```python
from build123d import *

# Parameters (mm, degrees)
RESSALTO_EXTRUS_O1_DEPTH = 22.5
CHANFRO1_SIZE            = 9
CORTE_EXTRUS_O1_REACH    = 24.5
ESBO_O3_W                = 1139.230904301
ESBO_O3_H                = 709.798033895
CORTE_EXTRUS_O5_DEPTH    = 1.5
ESBO_O5_R                = 3
CORTE_EXTRUS_O6_DEPTH    = 22
CORTE_EXTRUS_O8_DEPTH    = 10
CORTE_EXTRUS_O12_DEPTH   = 15
ESBO_O13_R               = 10.5
CORTE_EXTRUS_O13_DEPTH   = 5


with BuildPart() as part:
    # Esboço1 → Ressalto-extrusão1 (new body, symmetric)
    with BuildSketch(Plane.XY):
        with BuildLine():
            Line((-57.319579452, -8.082215343), (57.319579452, -8.082215343))
            Line((57.319579452, -8.082215343), (70, 2.557920862))
            Line((70, 2.557920862), (70, 117.296691049))
            ThreePointArc((70, 117.296691049), (70.546863139, 120.39810603), (72.121492792, 123.125444592))
            Line((72.121492792, 123.125444592), (112.878507208, 171.697762944))
            ThreePointArc((112.878507208, 171.697762944), (114.453136861, 174.425101506), (115, 177.526516487))
            Line((115, 177.526516487), (115, 237.712528581))
            ThreePointArc((115, 237.712528581), (114.396926208, 241.132730014), (112.660444431, 244.140404678))
            Line((112.660444431, 244.140404678), (75.567830361, 288.345660754))
            ThreePointArc((75.567830361, 288.345660754), (72.133568548, 290.980862527), (67.90738593, 291.917784657))
            Line((67.90738593, 291.917784657), (-67.90738593, 291.917784657))
            ThreePointArc((-67.90738593, 291.917784657), (-72.133568548, 290.980862527), (-75.567830361, 288.345660754))
            Line((-75.567830361, 288.345660754), (-112.660444431, 244.140404678))
            ThreePointArc((-112.660444431, 244.140404678), (-114.396926208, 241.132730014), (-115, 237.712528581))
            Line((-115, 237.712528581), (-115, 177.526516487))
            ThreePointArc((-115, 177.526516487), (-114.453136861, 174.425101506), (-112.878507208, 171.697762944))
            Line((-112.878507208, 171.697762944), (-72.121492792, 123.125444592))
            ThreePointArc((-72.121492792, 123.125444592), (-70.546863139, 120.39810603), (-70, 117.296691049))
            Line((-70, 117.296691049), (-70, 2.557920862))
            Line((-70, 2.557920862), (-57.319579452, -8.082215343))
        make_face()
        Polygon((-90, 175.546696324), (-90, 238.538123078), (-61.99113828, 271.917784657), (61.99113828, 271.917784657), (90, 238.538123078), (90, 175.546696324), (45, 121.917784657), (45, 11.917784657), (-45, 11.917784657), (-45, 121.917784657), align=None, mode=Mode.SUBTRACT)
    extrude(amount=RESSALTO_EXTRUS_O1_DEPTH, both=True)

    # Chanfro1
    chanfro1_edges = [part.edges().sort_by_distance(p)[0] for p in [
        (0, -8.082215343, 22.5),
        (63.659789726, -2.76214724, 22.5),
        (70, 59.927305955, 22.5),
        (70.546863139, 120.39810603, 22.5),
        (92.5, 147.411603768, 22.5),
        (114.453136861, 174.425101506, 22.5),
        (115, 207.619522534, 22.5),
        (114.396926208, 241.132730014, 22.5),
        (94.114137396, 266.243032716, 22.5),
        (72.133568548, 290.980862527, 22.5),
        (0, 291.917784657, 22.5),
        (-72.133568548, 290.980862527, 22.5),
        (-94.114137396, 266.243032716, 22.5),
        (-114.396926208, 241.132730014, 22.5),
        (-115, 207.619522534, 22.5),
        (-114.453136861, 174.425101506, 22.5),
        (-92.5, 147.411603768, 22.5),
        (-70.546863139, 120.39810603, 22.5),
        (-70, 59.927305955, 22.5),
        (-63.659789726, -2.76214724, 22.5),
    ]]
    chamfer(chanfro1_edges, length=CHANFRO1_SIZE)

    # Esboço3 → Corte-extrusão1 (cut, up to next)
    with BuildSketch(Plane.XY, mode=Mode.PRIVATE) as corte_extrus_o1_sk1:
        with Locations((-153.157436203, 152.53565808)):
            Rectangle(ESBO_O3_W, ESBO_O3_H)
    corte_extrus_o1_tool1 = extrude(corte_extrus_o1_sk1.sketch, amount=-CORTE_EXTRUS_O1_REACH, mode=Mode.PRIVATE) & part.part
    add(corte_extrus_o1_tool1.solids().sort_by_distance((-153.157436, 152.535658, 0))[0], mode=Mode.SUBTRACT)

    # Esboço4 → Corte-extrusão5 (cut)
    with BuildSketch(Plane.XY.offset(22.5)):
        Polygon((-60, 7.220997444), (-53.679877109, 1.917784657), (53.679877109, 1.917784657), (60, 7.220997444), (60, 125.792574104), (105, 179.421485771), (105, 237.712528581), (67.90738593, 281.917784657), (-67.90738593, 281.917784657), (-105, 237.712528581), (-105, 179.421485771), (-60, 125.792574104), align=None)
        Polygon((-90, 175.546696324), (-90, 238.538123078), (-61.99113828, 271.917784657), (61.99113828, 271.917784657), (90, 238.538123078), (90, 175.546696324), (45, 121.917784657), (45, 11.917784657), (-45, 11.917784657), (-45, 121.917784657), align=None, mode=Mode.SUBTRACT)
    extrude(amount=-CORTE_EXTRUS_O5_DEPTH, mode=Mode.SUBTRACT)

    # Esboço5 → Corte-extrusão6 (cut, through all)
    with BuildSketch(Plane.XY.offset(21)):
        with Locations((-93, 244)):
            Circle(ESBO_O5_R)
        with Locations((-52.5, 60.396230411)):
            Circle(ESBO_O5_R)
        with Locations((-73, 266.917784657)):
            Circle(ESBO_O5_R)
        with Locations((-52.5, 8.917784657)):
            Circle(ESBO_O5_R)
        with Locations((52.5, 8.917784657)):
            Circle(ESBO_O5_R)
        with Locations((73, 266.917784657)):
            Circle(ESBO_O5_R)
        with Locations((52.5, 60.396230411)):
            Circle(ESBO_O5_R)
        with Locations((93, 244)):
            Circle(ESBO_O5_R)
    extrude(amount=-CORTE_EXTRUS_O6_DEPTH, mode=Mode.SUBTRACT)

    # Esboço7 → Corte-extrusão8 (cut)
    with BuildSketch(Plane(origin=(0, 0, 0), x_dir=(-1, 0, 0), z_dir=(0, 0, -1))):
        Polygon((-73, 270.959236541), (-76.5, 268.938510599), (-76.5, 264.897058715), (-73, 262.876332773), (-69.5, 264.897058715), (-69.5, 268.938510599), align=None)
        Polygon((73, 270.959236541), (69.5, 268.938510599), (69.5, 264.897058715), (73, 262.876332773), (76.5, 264.897058715), (76.5, 268.938510599), align=None)
        Polygon((-93, 248.041451884), (-96.5, 246.020725942), (-96.5, 241.979274058), (-93, 239.958548116), (-89.5, 241.979274058), (-89.5, 246.020725942), align=None)
        Polygon((-52.5, 64.437682295), (-56, 62.416956353), (-56, 58.375504468), (-52.5, 56.354778526), (-49, 58.375504468), (-49, 62.416956353), align=None)
        Polygon((-52.5, 12.959236541), (-56, 10.938510599), (-56, 6.897058715), (-52.5, 4.876332773), (-49, 6.897058715), (-49, 10.938510599), align=None)
        Polygon((52.5, 12.959236541), (49, 10.938510599), (49, 6.897058715), (52.5, 4.876332773), (56, 6.897058715), (56, 10.938510599), align=None)
        Polygon((52.5, 64.437682295), (49, 62.416956353), (49, 58.375504468), (52.5, 56.354778526), (56, 58.375504468), (56, 62.416956353), align=None)
        Polygon((93, 248.041451884), (89.5, 246.020725942), (89.5, 241.979274058), (93, 239.958548116), (96.5, 241.979274058), (96.5, 246.020725942), align=None)
    extrude(amount=-CORTE_EXTRUS_O8_DEPTH, mode=Mode.SUBTRACT)

    # Esboço12 → Corte-extrusão12 (cut)
    with BuildSketch(Plane(origin=(0, 11.917784657, 0), x_dir=(1, 0, 0), z_dir=(0, 1, 0))):
        Polygon((-1.905573841, 14.34102327), (-11.457834044, 8.82602327), (-13.237834044, 5.742972833), (-13.237834044, -5.287027167), (-11.459750431, -8.366758325), (-1.915917658, -13.876892746), (1.640249569, -13.876892746), (11.220862954, -8.34552303), (12.986686363, -5.287027167), (12.986686363, 5.742972833), (11.206686363, 8.82602327), (1.654426159, 14.34102327), align=None)
    extrude(amount=-CORTE_EXTRUS_O12_DEPTH, mode=Mode.SUBTRACT)

    # Esboço13 → Corte-extrusão13 (cut)
    with BuildSketch(Plane.XZ.offset(8.082215343)):
        Circle(ESBO_O13_R)
    extrude(amount=-CORTE_EXTRUS_O13_DEPTH, mode=Mode.SUBTRACT)


solid = part.part
```
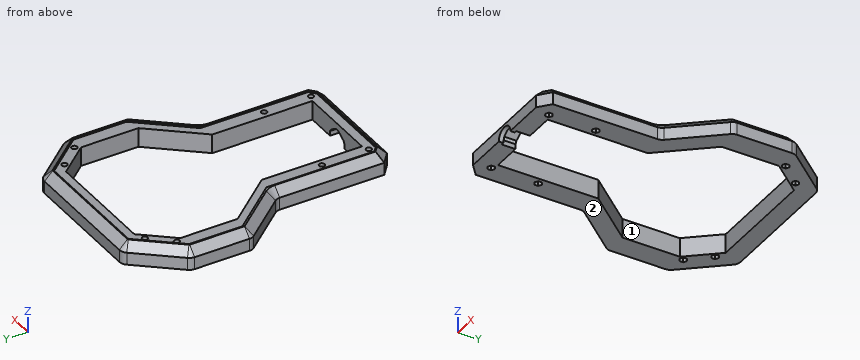
CAD build for the part. Positions are in the model's coordinates, mm. Face numbers are marked on the shaded views. Coordinates: 2 decimals unless noted, no trailing zeros. Write each loop counter-clockwise with the first axis right and the second up, starting at its lowest first coordinate (ties: lowest second). Pieces come first, ordered by that corner, then holes. Notation, with made-up numbers: (-10.5, 19.25) -> (10.5, 19.25) arc R10 ccw to (10.5, 38.25) -> close; hole circle Ø9 at (12, 84). An arc over 180 degrees is marked (long way). Return JSON: item names as keys, results as strings. Group by question number.
Q1. Pull direction X, two halves, no side cores. Call the marked faces 1 and 2: released by +X, released by -X, zero draft, split by the parting line, or undercut.
Q2. Drill centre lines: line 1 (X direction, y = 105, z = 13.25); line 2 (Y direction, x = -34, z = 12.5); line 3 (Y direction, x = -53, z = 5) (3 decimals). Where is each one in solid material? Low to high.
Q3. Cut at A-A, the plane y = 232.5. Give the cut face in (x, z), then the cut area to 3 significant figures.
Q4. Flat gauge pins, fed straight in: pin 1 (3 mm diameter, centred on y = 141.5, z = 15.5, fed in from -X); pin 2 (1.2 mm diameter, centred on y = 266.5, z = 6.5, fed in from -X); pin 3 (2 mm diameter, centred on y = 60, z = 7.5, fed in from +X). Where does each tip first touch, or does it go through?
Returned:
{
 "1": {"face 1": "undercut", "face 2": "zero draft"},
 "2": {"line 1": "x = -70 to -45, 45 to 70", "line 2": "y = -8.08 to 11.92, 271.92 to 291.92", "line 3": "y = -8.082 to 5.165, 12.671 to 56.643, 64.149 to 131.452, 271.918 to 291.918"},
 "3": {"outline": "(-115, 0) -> (-90, 0) -> (-90, 21) -> (-105, 21) -> (-105, 22.5) -> (-106, 22.5) -> (-115, 13.5) -> close; (90, 0) -> (115, 0) -> (115, 13.5) -> (106, 22.5) -> (105, 22.5) -> (105, 21) -> (90, 21) -> close", "area": "999 mm2"},
 "4": {"pin 1": "stops at x = -87.26", "pin 2": "stops at x = -94.4", "pin 3": "stops at x = 70"}
}
